```python
from build123d import *

# Parameters (mm, degrees)
SKETCH_1_W          = 72
SKETCH_1_H          = 62
EXTRUDE_1_DEPTH     = 2
SKETCH_2_W          = 18
SKETCH_2_H          = 2
CUT_EXTRUDE_1_DEPTH = 3
SKETCH_3_W          = 2
SKETCH_3_H          = 15.5
CUT_EXTRUDE_2_DEPTH = 3
SKETCH_4_W          = 36.5
SKETCH_4_H          = 16.955544823
SKETCH_4_W_2        = 51
SKETCH_4_H_2        = 12.596379679
SKETCH_4_H_3        = 9.075045386
CUT_EXTRUDE_3_DEPTH = 3


with BuildPart() as part:
    # ｽｹｯﾁ1 → ﾎﾞｽ - 押し出し1 (new body)
    with BuildSketch(Plane.XY):
        with Locations((-1.042641223, 9.736263736)):
            Rectangle(SKETCH_1_W, SKETCH_1_H)
    extrude(amount=EXTRUDE_1_DEPTH)

    # ｽｹｯﾁ2 → ｶｯﾄ - 押し出し1 (cut, through all)
    with BuildSketch(Plane.XY.offset(2)):
        with Locations((25.957358777, 39.736263736)):
            Rectangle(SKETCH_2_W, SKETCH_2_H)
        with Locations((-28.542641223, 39.736263736)):
            Rectangle(SKETCH_2_W, SKETCH_2_H)
        with Locations((-28.542641223, -20.263736264)):
            Rectangle(SKETCH_2_W, SKETCH_2_H)
        with Locations((25.957358777, -20.263736264)):
            Rectangle(SKETCH_2_W, SKETCH_2_H)
    extrude(amount=-CUT_EXTRUDE_1_DEPTH, mode=Mode.SUBTRACT)

    # ｽｹｯﾁ3 → ｶｯﾄ - 押し出し2 (cut, through all)
    with BuildSketch(Plane.XY.offset(2)):
        with Locations((33.957358777, 32.986263736)):
            Rectangle(SKETCH_3_W, SKETCH_3_H)
        with Locations((33.957358777, -13.513736264)):
            Rectangle(SKETCH_3_W, SKETCH_3_H)
        with Locations((-36.542641223, -13.513736264)):
            Rectangle(SKETCH_3_W, SKETCH_3_H)
        with Locations((-36.542641223, 32.986263736)):
            Rectangle(SKETCH_3_W, SKETCH_3_H)
    extrude(amount=-CUT_EXTRUDE_2_DEPTH, mode=Mode.SUBTRACT)

    # ｽｹｯﾁ4 → ｶｯﾄ - 押し出し3 (cut, through all)
    with BuildSketch(Plane.XY.offset(2)):
        with Locations((13.707358777, -9.261963853)):
            Rectangle(SKETCH_4_W, SKETCH_4_H)
        with Locations((-4.542641223, 13.634453576)):
            Rectangle(SKETCH_4_W_2, SKETCH_4_H_2)
        with Locations((-4.542641223, 30.673786429)):
            Rectangle(SKETCH_4_W_2, SKETCH_4_H_3)
    extrude(amount=-CUT_EXTRUDE_3_DEPTH, mode=Mode.SUBTRACT)


solid = part.part
```
Model file for the job. Use its own axes, mm. A direction names the side the tool comes from. Give positions to 0.01 mm unless a question says otherwise; leave off trailing zeros. Order: outer loops, then holes, each group sorted by start corner. A loop starts at its lowest first (then second) coordinate and runs counter-clockwise, first axis right, second up.
1) Wall check: probe 1 along Y at (x, z) = (12.5, 0.3); probe 2 along Y at (x, z) = (-9.5, 1.5); probe 3 along Y at (x, z) = (-24, 1.5). Give the ranges that are in metal, low to high.
2) Saw through at D-D, the plane x = -1. Write the cut outline in (y, z), then the cut area to 3 significant figures.
3) Saw through at C-C, the plane z = 1.4. Count the separate pieces of the cut face and the enclosed holes in it, then the cut area to 3 significant figures.
4) Mould opens along X. For faces 5 (the flat face through (-4.543, -9, 1)), 6 (the flat face through (34.957, 10, 1)), 7 (the flat face through (-37.043, 10, 1)) say: +X half, -X half, draft (parallel to the pull), parting line (faces both ways), or undercut.
5) Saw through at A-A, the plane x = -28.5. Write the cut outline in (y, z), then the cut area to 3 significant figures.
6) Saw through at B-B, the plane y = -5. Write the cut outline in (x, z), then the cut area to 3 significant figures.
7) 3-axis set-ups, long thin cutter, end or side, ignore diameter. For faces 1 (the flat face through (25, 38.736, 1)), 2 (the flat face through (20.957, 31, 1)), 3 (the flat face through (16.957, -20, 1)), 4 (the flat face through (-19.543, 40, 1)): which of +Z, -Z, +X, -X, +Y, -Y reach the whole face in a straight line?
8) Pin check, flat tips, straight feed: pin 1 (6 mm diameter, centred on x = 21, y = 33, fed in from -Z); pin 2 (0.6 mm diameter, centred on x = -28, z = 0.5, fed in from -Y); pin 3 (1 mm diameter, centred on y = -20.5, z = 1, fed in from +X); pin 4 (0.6 mm diameter, centred on y = 39.5, z = 1.5, fed in from -X). Stop position of each tip, or through.
Computed:
1. probe 1: y = -21.26 to -17.74, -0.78 to 7.34, 19.93 to 26.14, 35.21 to 40.74
1. probe 2: y = -21.26 to 7.34, 19.93 to 26.14, 35.21 to 40.74
1. probe 3: y = -19.26 to 7.34, 19.93 to 26.14, 35.21 to 38.74
2. outline: (-21.26, 0) - (-17.74, 0) - (-17.74, 2) - (-21.26, 2) - close; (-0.78, 0) - (7.34, 0) - (7.34, 2) - (-0.78, 2) - close; (19.93, 0) - (26.14, 0) - (26.14, 2) - (19.93, 2) - close; (35.21, 0) - (40.74, 0) - (40.74, 2) - (35.21, 2) - close
2. area: 46.7 mm2
3. separate pieces: 1
3. enclosed holes: 3
3. area: 2,500 mm2
4. face 5: undercut
4. face 6: +X half
4. face 7: -X half
5. outline: (-19.26, 0) - (7.34, 0) - (7.34, 2) - (-19.26, 2) - close; (19.93, 0) - (26.14, 0) - (26.14, 2) - (19.93, 2) - close; (35.21, 0) - (38.74, 0) - (38.74, 2) - (35.21, 2) - close
5. area: 72.7 mm2
6. outline: (-37.04, 0) - (-4.54, 0) - (-4.54, 2) - (-37.04, 2) - close; (31.96, 0) - (34.96, 0) - (34.96, 2) - (31.96, 2) - close
6. area: 71.0 mm2
7. face 1: +Z, -Z, +X, +Y
7. face 2: +Z, -Z
7. face 3: +Z, -Z, +X, -Y
7. face 4: +Z, -Z, -X, +Y
8. pin 1: stops at z = 0
8. pin 2: stops at y = -19.26
8. pin 3: stops at x = 16.96
8. pin 4: stops at x = -19.54
